Could you check a few things on this model? Use its own coordinates, in mm. A direction names the side the tool comes from. Give positions to 0.01 mm unless a question says otherwise; leave off trailing zeros. Order: outer loops, then holes, each group sorted by start corner. A loop starts at its lowest first (then second) coordinate and runs counter-clockwise, first axis right, second up. Notation, with made-up numbers: M -15,10 L 40,10 A36 ccw 40,49 Z; hole C -23.5,46.5 d5. An arc over 180 degrees is marked long. Answer in a Markdown table with one row per item. Add a question column.
Autodesk Inventor part; units mm, degrees
ref_plane "YZ Plane" through (0, 0, 0) normal (1, 0, 0) x (0, 1, 0)
ref_plane "XZ Plane" through (0, 0, 0) normal (0, 1, 0) x (-1, 0, 0)
ref_plane "XY Plane" through (0, 0, 0) normal (0, 0, 1) x (1, 0, 0)
sketch "Sketch1" plane through (0, 0, 0) normal (1, 0, 0) x (0, 1, 0)
  line L0 (-46, -7.5) -> (-46, 1)
  line L1 (-42, 5) -> (42, 5)
  line L2 (46, 1) -> (46, -7.5)
  line L3 (-41, -12.5) -> (-39.95, -12.5)
  line L4 (-40.25, -2.509) -> (-40.25, 0)
  line L5 (-40.25, 0) -> (40.25, 0)
  line L6 (-1, 5) -> (-1, 13)
  line L7 (-1, 13) -> (1, 13)
  line L8 (1, 13) -> (1, 5)
  line L9 (-46, 19) -> (46, 19)
  line L10 (46, 19) -> (46, 13)
  line L11 (46, 13) -> (-46, 13)
  line L12 (-46, 13) -> (-46, 19)
  arc A0 (46, 1) -> (42, 5) centre (42, 1) ccw
  arc A1 (-42, 5) -> (-46, 1) centre (-42, 1) ccw
  arc A2 (40.25, 0) -> (33.25, 0) centre (36.75, 0) ccw
  arc A3 (-33.25, 0) -> (-40.25, 0) centre (-36.75, 0) ccw
  line L13 (40.25, 0) -> (40.25, -2.509)
  arc A4 (-39.95, -12.5) -> (-40.25, -2.509) centre (-39.95, -7.5) ccw
  arc A5 (-46, -7.5) -> (-41, -12.5) centre (-41, -7.5) ccw
  circle A6 centre (39.95, -7.5) radius 5
  line L14 (41, -12.5) -> (39.95, -12.5)
  arc A7 (41, -12.5) -> (46, -7.5) centre (41, -7.5) ccw
  point P0 (0, 0)
  point P1 (-46, -12.5)
  point P2 (-46, 5)
  point P3 (46, 5)
  point P4 (46, -12.5)
  point P5 (0, 5)
  point P6 (0, 0)
  point P7 (0, 13)
  point P8 (1, 13)
  point P9 (-1, 13)
  point P10 (-40.25, -1.2545)
  point P11 (40.25, -1.2545)
  point P12 (40.25, -2.509)
  dimension "d71" = 10
  dimension "d2" = 80.5
  dimension "d10" = 92
  dimension "d11" = 5
  dimension "d13" = 2
  dimension "d14" = 8
  dimension "d15" = 6
  dimension "d52" = 4
  dimension "d53" = 7
  dimension "d54" = 7
  dimension "d67" = 10
  dimension "d68" = 7.5
  dimension "d69" = 0.3
  dimension "d70" = 5
  dimension "d72" = 0.3
  dimension "d73" = 5
extrude "Extrusion1" add sketch "Sketch1" along normal mid plane 50 contours L0 A1 L1 A0 L2 A7 L14 A6 L13 A2 L5 A3 L4 A4 L3 A5 | L6 L7 L8 L1 | L11 L12 L9 L10 L7 | A6
sketch "Sketch2" plane through (-25, -46, 19) normal (0, 0, 1) x (1, 0, 0)
  line L0 (0, 0) -> (50, 0)
  line L1 (50, 92) -> (50, 0)
  line L2 (0, 92) -> (50, 92)
  line L3 (0, 0) -> (0, 92)
  line L4 (25.625, 10) -> (24.375, 10)
  line L5 (24.375, 10) -> (24.375, 82)
  line L6 (24.375, 82) -> (25.625, 82)
  line L7 (25.625, 82) -> (25.625, 10)
  line L8 (25.625, 10) -> (24.375, 82) construction
  line L9 (24.375, 10) -> (25.625, 82) construction
  point P0 (25, 46)
  point P1 (20.75, 0)
  point P2 (20.75, 50)
  point P3 (19.25, 50)
  point P4 (19.25, 0)
  point P5 (25, 10)
  dimension "d16" = 1.25
  dimension "d19" = 10
extrude "Extrusion2" add sketch "Sketch2" along normal blind 8 contours L4 L5 L6 L7
sketch "Sketch3" plane through (-25, -46, 19) normal (0, 0, 1) x (1, 0, 0)
  line L0 (25.625, 82) -> (25.625, 10)
  line L1 (25.625, 10) -> (24.375, 10)
  line L2 (24.375, 10) -> (24.375, 82)
  line L3 (24.375, 82) -> (25.625, 82)
  line L4 (0, 0) -> (50, 0)
  line L5 (50, 92) -> (50, 0)
  line L6 (0, 92) -> (50, 92)
  line L7 (0, 0) -> (0, 92)
  line L8 (25.625, 10) -> (24.375, 10)
  line L9 (25, 10) -> (25, 0)
  line L10 (24.375, 82) -> (25.625, 82)
  line L11 (25, 82) -> (25, 92)
  point P0 (25, 46)
  point P1 (25, 5)
  point P2 (25, 87)
hole "Hole1" at (0, -41, 19) at (0, 41, 19) direction (0, 0, -1) diameter 4 depth 8 tip angle 118
sketch "Sketch4" plane through (-25, -46, 27) normal (0, 0, 1) x (1, 0, 0)
  line L0 (0, 10) -> (50, 10)
  line L1 (50, 10) -> (50, 82)
  line L2 (50, 82) -> (0, 82)
  line L3 (0, 82) -> (0, 10)
  line L4 (0, 10) -> (50, 82) construction
  line L5 (50, 10) -> (0, 82) construction
  line L6 (25.625, 82) -> (24.375, 82)
  line L7 (0, 0) -> (0, 92)
  point P0 (25, 46)
  point P1 (25, 82)
  point P2 (0, 46)
extrude "Extrusion3" add sketch "Sketch4" along normal blind 6
sketch "Sketch5" plane through (-25, -46, 33) normal (0, 0, 1) x (1, 0, 0)
  line L0 (50, 82) -> (0, 82)
  line L1 (0, 82) -> (0, 10)
  line L2 (0, 10) -> (50, 10)
  line L3 (50, 10) -> (50, 82)
  line L4 (5, 46) -> (45, 46)
  point P0 (25, 46)
  point P1 (25, 46)
  dimension "d29" = 5
hole "Hole2" at (-20, 0, 33) at (20, 0, 33) direction (0, 0, -1) diameter 4 depth 8 tip angle 118
sketch "Sketch6" plane through (-25, -46, 33) normal (0, 0, 1) x (1, 0, 0)
  circle A0 centre (5, 46) radius 2
  circle A1 centre (45, 46) radius 2
  line L0 (50, 82) -> (0, 82)
  line L1 (0, 82) -> (0, 10)
  line L2 (0, 10) -> (50, 10)
  line L3 (50, 10) -> (50, 82)
  line L4 (25, 16) -> (25, 76)
  point P0 (25, 46)
  point P1 (25, 46)
  point P2 (25, 46)
  dimension "d38" = 60
hole "Hole3" at (0, -30, 33) at (0, 30, 33) direction (0, 0, -1) diameter 4 depth 5
chamfer "Chamfer1" distance 5 angle 45 4 edges at (-25, -46, 16) (-25, 46, 16) (25, -46, 16) (25, 46, 16)
chamfer "Chamfer2" distance 8 angle 45 4 edges at (25, 36, 30) (25, -36, 30) (-25, -36, 30) (-25, 36, 30)
fillet "Fillet1" radius 2 6 edges at (0.625, 0, 19) (-0.625, 0, 19) (0, -1, 5) (0, 1, 5) (0, -1, 13) (0, 1, 13)
properties part number "Rail-FlextureBaseLarge" material "ABS Plastic"
1. For faces 4 (the flat face through (21, -32, 30)), 5 (the cylindrical face through (-0.35, -1.57, 5.6)), 6 (the cylindrical face through (1.195, -0.504, 19.601)), which set-ups out of +Z, -Z, +X, -X, +Y, -Y let a thin tool reach every point of the face, with its end or its side?
2. Suppose I cut it at C-C on y = 30. List the corners of the cut face in (x, z) for me (3 decimals), plus the area to 3 significant figures.
3. Suppose I cut it at A-A on y = -18. List the corners of the cut face in (x, z) for me (3 decimals).
4. If I drill on line 1 along Z through (x, y) = (11, -20); line 2 along X through (y, z) = (0, 31); line 3 along Y through (x, z) = (0, 29.65), over which ranges is the centre line in solid material (lowest first)? Write a range as [from, to].
5. Thinking about a two-plate mould opening in X: for faces 1 (the flat face through (-23, -43, 16)), 2 (the cylindrical face through (-0.35, -44.5, -11.07)), 3 (the cylindrical face through (18, 0, 30)), which applies, pulls with the +X half, pulls with the -X half, needs draft (parallel to the pull), parting line crosses it, or undercut?
6. Suppose I cut it at D-D on z = 8.5. List the corners of the cut face in (x, y) for me, plus the area to 3 significant figures.
7. Will these pins go through, and if not, where does the flat tip stop? P1, Ø12, axis at x = -16, y = -12.5, coming from the -Z side; P2, Ø7, axis at x = 8.5, z = 26.5, coming from the +Y side; P3, Ø1.2, axis at x = 0.5, y = 30, coming from the +Z side.
Findings below:
| question | item | result |
|---|---|---|
| 1 | face 4 | +Z, +X, -Y |
| 1 | face 5 | +X, -X, -Y |
| 1 | face 6 | +X, +Y, -Y |
| 2 | outline | M -25,0 L 25,0 L 25,5 L -25,5 Z; M -25,13 L 25,13 L 25,19 L 2.625,19 A2 cw 0.625,21 L 0.625,27 L 23,27 L 23,33 L 2,33 L 2,28 L -2,28 L -2,33 L -23,33 L -23,27 L -0.625,27 L -0.625,21 A2 cw -2.625,19 L -25,19 Z |
| 2 | area | 818 mm2 |
| 3 | outline | M -25,0 L 25,0 L 25,5 L -25,5 Z; M -25,13 L 25,13 L 25,19 L 2.625,19 A2 cw 0.625,21 L 0.625,27 L 25,27 L 25,33 L -25,33 L -25,27 L -0.625,27 L -0.625,21 A2 cw -2.625,19 L -25,19 Z |
| 4 | line 1 | [0, 5], [13, 19], [27, 33] |
| 4 | line 2 | [-25, -22], [-18, 18], [22, 25] |
| 4 | line 3 | [-36, -32], [-28, 28], [32, 36] |
| 5 | face 1 | pulls with the -X half |
| 5 | face 2 | needs draft |
| 5 | face 3 | undercut |
| 6 | outline | M -25,-1 L 25,-1 L 25,1 L -25,1 Z |
| 6 | area | 100 mm2 |
| 7 | P1 | z = 0 |
| 7 | P2 | y = 36 |
| 7 | P3 | z = 28 |
